Read the model definition and answer for the solid it produces. Units are mm, in the model's axes. A direction names the side the tool comes from. Coordinates: 2 decimals unless noted, no trailing zeros. Write each loop counter-clockwise with the first axis right and the second up, starting at its lowest first coordinate (ties: lowest second). Pieces come first, ordered by that corner, then holes. Notation, with made-up numbers: (82, 41) -> (120, 41) arc R21 cw to (120, 60) -> close; hole circle Ø5 at (4.5, 30). An arc over 180 degrees is marked (long way). Write item = value, one per line. Start each with the question number.
1) Find the intervals of material crossed by line 1 along X through (y, z) = (-18.1, 0); line 2 along Z through (x, y) = (0, -25); line 3 along Z through (x, y) = (0, -20.5), in increasing order. Write a range as from..to.
2) For a pull along Z with two mould halves and no side action, classify faces 5 (the face through (-13.24, -8.69, 4.17)), 6 (the face through (-13.1, -17.63, -5.2)), 7 (the face through (-3, -18.97, -9)) as released by +Z, released by -Z, zero draft, split by the parting line, or undercut.
3) A tool of negligible diameter and unlimited length cuts with its end or side. For faces 1 (the face through (5.2, -17.63, 13.1)), 2 (the face through (5, -18.74, 7.84)), 3 (the face through (5, -26.34, 7.84)), 4 (the face through (13.04, -17.63, -5.25)), from which of +Z, -Z, +X, -X, +Y, -Y can it reach the whole face along a straight path? Write none if from no direction.
4) Section A-A (x = 6.25) is taken. Determine the outline of the cut face in (y, z).
5) Section D-D (y = -16.5) is taken. Determine the outline of the cut face in (x, z), plus the area to 3 significant figures.
6) Section B-B (z = -4.25) is taken. Determine the outline of the cut face in (x, y), plus the area to 3 significant figures.
7) Flat-ended cylindrical pins translate along their axes: pin 1 Ø4.5 at (x, z) = (-3, 11) entering from -Y; pin 2 Ø1.2 at (x, z) = (-12, -5) entering from -Y; pin 3 Ø2 at (x, z) = (-3.5, 4.5) entering from +Y; pin 4 Ø9.5 at (x, z) = (-3, 3.5) entering from +Y. Find the tip coordinate at first contact, or state that the pin passes through.
8) Section C-C (y = -24) is taken. Determine the outline of the cut face in (x, z).
Autodesk Inventor part; units mm, degrees
ref_plane "Plano de trabajo2" through (0, -18.5, 0) normal (0, 1, 0) x (1, 0, 0)
ref_plane "YZ Plane" through (0, 0, 0) normal (1, 0, 0) x (0, 1, 0)
ref_plane "XZ Plane" through (0, 0, 0) normal (0, 1, 0) x (-1, 0, 0)
sketch "Boceto1" plane through (0, 0, 0) normal (0, 1, 0) x (-1, 0, 0)
  circle A0 centre (0, 0) radius 10.7
  circle A1 centre (0, 0) radius 13.88
  dimension "d0" = 21.4
  dimension "d1" = 27.76
extrude "Extrusión1" add sketch "Boceto1" against normal blind 23.6
sketch "Boceto2" plane through (0, -23.6, 0) normal (0, -1, 0) x (1, 0, 0)
  circle A0 centre (0, 0) radius 13.88
  line L0 (0, -13.88) -> (-5.75, -13.88)
  line L1 (0, -13.88) -> (5.75, -13.88)
  line L2 (13.88, 0) -> (13.88, -5.75)
  line L3 (13.88, 0) -> (13.88, 5.75)
  line L4 (0, 13.88) -> (5.75, 13.88)
  line L5 (0, 13.88) -> (-5.75, 13.88)
  line L6 (-13.88, 0) -> (-13.88, -5.75)
  line L7 (-13.88, 0) -> (-13.88, 5.75)
  line L8 (-13.88, 5.75) -> (-5.75, 13.88)
  line L9 (5.75, 13.88) -> (13.88, 5.75)
  line L10 (13.88, -5.75) -> (5.75, -13.88)
  line L11 (-5.75, -13.88) -> (-13.88, -5.75)
  dimension "d5" = 5.75
  dimension "d6" = 5.75
  dimension "d7" = 5.75
  dimension "d8" = 5.75
  dimension "d9" = 5.75
  dimension "d10" = 5.75
  dimension "d11" = 5.75
  dimension "d12" = 5.75
extrude "Extrusión2" add sketch "Boceto2" against normal blind 5.97
ref_plane "Plano de trabajo2" through (0, -18.5, 0) normal (0, 1, 0) x (1, 0, 0)
sketch "Boceto4" plane through (0, -18.5, 0) normal (0, 1, 0) x (1, 0, 0)
  circle A0 centre (0, 0) radius 6.8
  dimension "d18" = 13.6
extrude "Extrusión4" add sketch "Boceto4" against normal blind 18.97
sketch "Boceto5" plane through (0, 0, 0) normal (0, 1, 0) x (1, 0, 0)
  circle A0 centre (0, 0) radius 10.7
extrude "Extrusión5" cut sketch "Boceto5" against normal blind 18.97
sketch "Boceto6" plane through (0, -37.47, 0) normal (0, -1, 0) x (1, 0, 0)
  circle A0 centre (0, 0) radius 6.7
  circle A1 centre (0, 0) radius 9.3
  dimension "d25" = 13.4
  dimension "d26" = 18.6
extrude "Extrusión6" add sketch "Boceto6" against normal blind 18.97
sketch "Boceto7" plane through (0, -37.47, 0) normal (0, -1, 0) x (1, 0, 0)
  circle A0 centre (0, 0) radius 6.8
  dimension "d29" = 13.6
extrude "Extrusión7" cut sketch "Boceto7" against normal blind 18.97
thread "Rosca2"
sketch "Boceto9" plane through (0, -37.47, 0) normal (0, -1, 0) x (1, 0, 0)
  circle A0 centre (0, 0) radius 9.3
extrude "Extrusión8" cut sketch "Boceto9" against normal blind 8.47
properties part number "Acople con rosca" material "PVC, no plastificado"
Answer key:
q1.line_1 = -13.88..-10.7, 10.7..13.88
q1.line_2 = -9.3..-6.8, 6.8..9.3
q1.line_3 = -13.88..-6.8, 6.8..13.88
q2.face_5 = split by the parting line
q2.face_6 = zero draft
q2.face_7 = undercut
q3.face_1 = +Z, +X, +Y
q3.face_2 = +Y
q3.face_3 = -Y
q3.face_4 = -Z, +X, +Y
q4.outline = (-29, -6.89) -> (-23.6, -6.89) -> (-23.6, -13.38) -> (-17.63, -13.38) -> (-17.63, -12.39) -> (0, -12.39) -> (0, -8.68) -> (-18.97, -8.68) -> (-18.97, -6.89) -> (-18.5, -6.89) -> (-18.5, -2.68) -> (-29, -2.68) -> close; (-29, 2.68) -> (-18.5, 2.68) -> (-18.5, 6.89) -> (-18.97, 6.89) -> (-18.97, 8.68) -> (0, 8.68) -> (0, 12.39) -> (-17.63, 12.39) -> (-17.63, 13.38) -> (-23.6, 13.38) -> (-23.6, 6.89) -> (-29, 6.89) -> close
q5.outline = circle Ø27.76 at (0, 0); hole circle Ø21.4 at (0, 0)
q5.area = 246 mm^2
q6.outline = (-13.88, -23.6) -> (-8.27, -23.6) -> (-8.27, -29) -> (-5.31, -29) -> (-5.31, -18.5) -> (-8.27, -18.5) -> (-8.27, -18.97) -> (-9.82, -18.97) -> (-9.82, 0) -> (-13.21, 0) -> (-13.21, -17.63) -> (-13.88, -17.63) -> close; (5.31, -29) -> (8.27, -29) -> (8.27, -23.6) -> (13.88, -23.6) -> (13.88, -17.63) -> (13.21, -17.63) -> (13.21, 0) -> (9.82, 0) -> (9.82, -18.97) -> (8.27, -18.97) -> (8.27, -18.5) -> (5.31, -18.5) -> close
q6.area = 245 mm^2
q7.pin_1 = -29
q7.pin_2 = -23.6
q7.pin_3 = through
q7.pin_4 = -18.5
q8.outline = circle Ø18.6 at (0, 0); hole circle Ø13.6 at (0, 0)
